from build123d import *
from OCP.BRepFilletAPI import BRepFilletAPI_MakeChamfer

# Parameters (mm, degrees)
SKETCH_1_R      = 1.55
EXTRUDE_1_DEPTH = 2.5
FILLET_1_R      = 10
CHAMFER_2_SIZE  = 0.615
CHAMFER_2_SIZE2 = 0.355070416


with BuildPart() as part:
    # 草图1 → 凸台-拉伸1 (new body)
    with BuildSketch(Plane(origin=(0, 0, 0), x_dir=(1, 0, 0), z_dir=(0, 1, 0))):
        with BuildLine():
            Line((47.899982554, 52.633397656), (59.52497064, 26.588251477))
            Line((59.52497064, 26.588251477), (85.869588061, 26.588251477))
            Line((85.869588061, 26.588251477), (94.505759306, 0))
            Line((94.505759306, 0), (85.869588061, -26.588251477))
            Line((85.869588061, -26.588251477), (59.52497064, -26.588251477))
            Line((59.52497064, -26.588251477), (47.899982554, -52.633397656))
            ThreePointArc((47.899982554, -52.633397656), (43.362068791, -56.315801292), (37.709796983, -54.831018053))
            ThreePointArc((37.709796983, -54.831018053), (34.400449937, -52.764318952), (30.978168019, -50.89055015))
            Line((30.978168019, -50.89055015), (-30.978168019, -50.89055015))
            ThreePointArc((-30.978168019, -50.89055015), (-34.400449937, -52.764318952), (-37.709796983, -54.831018053))
            ThreePointArc((-37.709796983, -54.831018053), (-43.362068791, -56.315801292), (-47.899982554, -52.633397656))
            Line((-47.899982554, -52.633397656), (-59.52497064, -26.588251477))
            Line((-59.52497064, -26.588251477), (-85.869588061, -26.588251477))
            Line((-85.869588061, -26.588251477), (-94.505759306, 0))
            Line((-94.505759306, 0), (-85.869588061, 26.588251477))
            Line((-85.869588061, 26.588251477), (-59.52497064, 26.588251477))
            Line((-59.52497064, 26.588251477), (-47.899982554, 52.633397656))
            ThreePointArc((-47.899982554, 52.633397656), (-43.362068791, 56.315801292), (-37.709796983, 54.831018053))
            ThreePointArc((-37.709796983, 54.831018053), (-34.400449937, 52.764318952), (-30.978168019, 50.89055015))
            Line((-30.978168019, 50.89055015), (30.978168019, 50.89055015))
            ThreePointArc((30.978168019, 50.89055015), (34.400449937, 52.764318952), (37.709796983, 54.831018053))
            ThreePointArc((37.709796983, 54.831018053), (43.362068791, 56.315801292), (47.899982554, 52.633397656))
        make_face()
        with Locations(Location((42, 50, 0), (0, 0, 270))):
            Circle(SKETCH_1_R, mode=Mode.SUBTRACT)
        with Locations(Location((42, -50, 0), (0, 0, 90))):
            Circle(SKETCH_1_R, mode=Mode.SUBTRACT)
        with Locations(Location((-42, -50, 0), (0, 0, 270))):
            Circle(SKETCH_1_R, mode=Mode.SUBTRACT)
        with Locations(Location((-42, 50, 0), (0, 0, 90))):
            Circle(SKETCH_1_R, mode=Mode.SUBTRACT)
        with Locations(Location((36, 43, 0), (0, 0, 270))):
            Circle(SKETCH_1_R, mode=Mode.SUBTRACT)
        with Locations(Location((32, -42, 0), (0, 0, 270))):
            Circle(SKETCH_1_R, mode=Mode.SUBTRACT)
        with Locations(Location((-32, -42, 0), (0, 0, 90))):
            Circle(SKETCH_1_R, mode=Mode.SUBTRACT)
        with Locations(Location((-36, 43, 0), (0, 0, 90))):
            Circle(SKETCH_1_R, mode=Mode.SUBTRACT)
        with Locations(Location((70.5, 9.435839055, 0), (0, 0, 270))):
            Circle(SKETCH_1_R, mode=Mode.SUBTRACT)
        with Locations(Location((70.5, -9.435839055, 0), (0, 0, 90))):
            Circle(SKETCH_1_R, mode=Mode.SUBTRACT)
        with Locations(Location((-70.5, -9.435839055, 0), (0, 0, 270))):
            Circle(SKETCH_1_R, mode=Mode.SUBTRACT)
        with Locations(Location((-70.5, 9.435839055, 0), (0, 0, 90))):
            Circle(SKETCH_1_R, mode=Mode.SUBTRACT)
        with Locations(Location((87.3, 0, 0), (0, 0, 270))):
            Circle(SKETCH_1_R, mode=Mode.SUBTRACT)
        with Locations(Location((-87.3, 0, 0), (0, 0, 90))):
            Circle(SKETCH_1_R, mode=Mode.SUBTRACT)
        with BuildLine():
            Line((77.169642998, -17.5), (77.169642998, 17.5))
            ThreePointArc((77.169642998, 17.5), (79.669642998, 20), (82.169642998, 17.5))
            Line((82.169642998, 17.5), (82.169642998, -17.5))
            ThreePointArc((82.169642998, -17.5), (79.669642998, -20), (77.169642998, -17.5))
        make_face(mode=Mode.SUBTRACT)
        with BuildLine():
            Line((-77.169642998, -17.5), (-77.169642998, 17.5))
            ThreePointArc((-77.169642998, 17.5), (-79.669642998, 20), (-82.169642998, 17.5))
            Line((-82.169642998, 17.5), (-82.169642998, -17.5))
            ThreePointArc((-82.169642998, -17.5), (-79.669642998, -20), (-77.169642998, -17.5))
        make_face(mode=Mode.SUBTRACT)
        with BuildLine():
            Line((-24.995975583, 14.429581723), (-10.56639386, 0))
            Line((-10.56639386, 0), (-24.995975583, -14.429581723))
            ThreePointArc((-24.995975583, -14.429581723), (-27.869597938, -17.042325553), (-30.978168019, -19.370614155))
            ThreePointArc((-30.978168019, -19.370614155), (-28.024295248, 0), (-30.978168019, 19.370614155))
            ThreePointArc((-30.978168019, 19.370614155), (-27.869597938, 17.042325553), (-24.995975583, 14.429581723))
        make_face(mode=Mode.SUBTRACT)
        with BuildLine():
            Line((14.429581723, 24.995975583), (0, 10.56639386))
            Line((0, 10.56639386), (-14.429581723, 24.995975583))
            ThreePointArc((-14.429581723, 24.995975583), (-17.042325553, 27.869597938), (-19.370614155, 30.978168019))
            ThreePointArc((-19.370614155, 30.978168019), (0, 28.024295248), (19.370614155, 30.978168019))
            ThreePointArc((19.370614155, 30.978168019), (17.042325553, 27.869597938), (14.429581723, 24.995975583))
        make_face(mode=Mode.SUBTRACT)
        with BuildLine():
            Line((24.995975583, -14.429581723), (10.56639386, 0))
            Line((10.56639386, 0), (24.995975583, 14.429581723))
            ThreePointArc((24.995975583, 14.429581723), (27.869597938, 17.042325553), (30.978168019, 19.370614155))
            ThreePointArc((30.978168019, 19.370614155), (28.024295248, 0), (30.978168019, -19.370614155))
            ThreePointArc((30.978168019, -19.370614155), (27.869597938, -17.042325553), (24.995975583, -14.429581723))
        make_face(mode=Mode.SUBTRACT)
        with BuildLine():
            Line((-14.429581723, -24.995975583), (0, -10.56639386))
            Line((0, -10.56639386), (14.429581723, -24.995975583))
            ThreePointArc((14.429581723, -24.995975583), (17.042325553, -27.869597938), (19.370614155, -30.978168019))
            ThreePointArc((19.370614155, -30.978168019), (0, -28.024295248), (-19.370614155, -30.978168019))
            ThreePointArc((-19.370614155, -30.978168019), (-17.042325553, -27.869597938), (-14.429581723, -24.995975583))
        make_face(mode=Mode.SUBTRACT)
        with BuildLine():
            Line((41.468701347, -26.829343455), (41.468701347, 26.829343455))
            ThreePointArc((41.468701347, 26.829343455), (44.919200659, 30.279842767), (48.36969997, 26.829343455))
            Line((48.36969997, 26.829343455), (48.36969997, -26.829343455))
            ThreePointArc((48.36969997, -26.829343455), (44.919200659, -30.279842767), (41.468701347, -26.829343455))
        make_face(mode=Mode.SUBTRACT)
        with BuildLine():
            Line((-26.453510137, -34.636976429), (26.453510137, -34.636976429))
            ThreePointArc((26.453510137, -34.636976429), (29.060662927, -37.244129219), (26.453510137, -39.851282009))
            Line((26.453510137, -39.851282009), (-26.453510137, -39.851282009))
            ThreePointArc((-26.453510137, -39.851282009), (-29.060662927, -37.244129219), (-26.453510137, -34.636976429))
        make_face(mode=Mode.SUBTRACT)
        with BuildLine():
            Line((-26.453510137, 34.636976429), (26.453510137, 34.636976429))
            ThreePointArc((26.453510137, 34.636976429), (29.060662927, 37.244129219), (26.453510137, 39.851282009))
            Line((26.453510137, 39.851282009), (-26.453510137, 39.851282009))
            ThreePointArc((-26.453510137, 39.851282009), (-29.060662927, 37.244129219), (-26.453510137, 34.636976429))
        make_face(mode=Mode.SUBTRACT)
        with BuildLine():
            Line((-41.468701347, -26.829343455), (-41.468701347, 26.829343455))
            ThreePointArc((-41.468701347, 26.829343455), (-44.919200659, 30.279842767), (-48.36969997, 26.829343455))
            Line((-48.36969997, 26.829343455), (-48.36969997, -26.829343455))
            ThreePointArc((-48.36969997, -26.829343455), (-44.919200659, -30.279842767), (-41.468701347, -26.829343455))
        make_face(mode=Mode.SUBTRACT)
    extrude(amount=EXTRUDE_1_DEPTH)

    # 圆角1
    fillet_1_edges = [part.edges().sort_by_distance(p)[0] for p in [
        (59.52497064, 1.25, -26.588251477),
        (85.869588061, 1.25, -26.588251477),
        (94.505759306, 1.25, 0),
        (85.869588061, 1.25, 26.588251477),
        (59.52497064, 1.25, 26.588251477),
        (30.978168019, 1.25, 50.89055015),
        (-30.978168019, 1.25, 50.89055015),
        (-59.52497064, 1.25, 26.588251477),
        (-85.869588061, 1.25, 26.588251477),
        (-94.505759306, 1.25, 0),
        (-85.869588061, 1.25, -26.588251477),
        (-59.52497064, 1.25, -26.588251477),
        (-30.978168019, 1.25, -50.89055015),
        (30.978168019, 1.25, -50.89055015),
    ]]
    fillet(fillet_1_edges, radius=FILLET_1_R)

    # 倒角2: one chamfer whose edges measure the first distance from different faces: ONE call of the kernel's chamfer builder (chamfer() names one face for all edges)
    chamfer_2_edges_1 = [part.edges().sort_by_distance(p)[0] for p in [
        (70.5, 0, 10.985839055),
    ]]
    chamfer_2_side_1 = [part.faces().sort_by_distance(p)[0] for p in [
        (70.5, 1.25, 10.985839055),
    ]]
    chamfer_2_edges_2 = [part.edges().sort_by_distance(p)[0] for p in [
        (-70.5, 0, 7.885839055),
    ]]
    chamfer_2_side_2 = [part.faces().sort_by_distance(p)[0] for p in [
        (-70.5, 1.25, 7.885839055),
    ]]
    chamfer_2_edges_3 = [part.edges().sort_by_distance(p)[0] for p in [
        (70.5, 0, -10.985839055),
    ]]
    chamfer_2_side_3 = [part.faces().sort_by_distance(p)[0] for p in [
        (70.5, 1.25, -10.985839055),
    ]]
    chamfer_2_edges_4 = [part.edges().sort_by_distance(p)[0] for p in [
        (-70.5, 0, -7.885839055),
    ]]
    chamfer_2_side_4 = [part.faces().sort_by_distance(p)[0] for p in [
        (-70.5, 1.25, -7.885839055),
    ]]
    chamfer_2_edges_5 = [part.edges().sort_by_distance(p)[0] for p in [
        (87.3, 0, -1.55),
    ]]
    chamfer_2_side_5 = [part.faces().sort_by_distance(p)[0] for p in [
        (87.3, 1.25, -1.55),
    ]]
    chamfer_2_edges_6 = [part.edges().sort_by_distance(p)[0] for p in [
        (-87.3, 0, 1.55),
    ]]
    chamfer_2_side_6 = [part.faces().sort_by_distance(p)[0] for p in [
        (-87.3, 1.25, 1.55),
    ]]
    chamfer_2_edges_7 = [part.edges().sort_by_distance(p)[0] for p in [
        (-42, 0, 48.45),
    ]]
    chamfer_2_side_7 = [part.faces().sort_by_distance(p)[0] for p in [
        (-42, 1.25, 48.45),
    ]]
    chamfer_2_edges_8 = [part.edges().sort_by_distance(p)[0] for p in [
        (-42, 0, -48.45),
    ]]
    chamfer_2_side_8 = [part.faces().sort_by_distance(p)[0] for p in [
        (-42, 1.25, -48.45),
    ]]
    chamfer_2_edges_9 = [part.edges().sort_by_distance(p)[0] for p in [
        (42, 0, -51.55),
    ]]
    chamfer_2_side_9 = [part.faces().sort_by_distance(p)[0] for p in [
        (42, 1.25, -51.55),
    ]]
    chamfer_2_edges_10 = [part.edges().sort_by_distance(p)[0] for p in [
        (42, 0, 51.55),
    ]]
    chamfer_2_side_10 = [part.faces().sort_by_distance(p)[0] for p in [
        (42, 1.25, 51.55),
    ]]
    chamfer_2 = BRepFilletAPI_MakeChamfer(part.part.solid().wrapped)
    for e in chamfer_2_edges_1:
        chamfer_2.Add(CHAMFER_2_SIZE, CHAMFER_2_SIZE2, e.wrapped, chamfer_2_side_1[0].wrapped)  # the first distance lies on this face
    for e in chamfer_2_edges_2:
        chamfer_2.Add(CHAMFER_2_SIZE, CHAMFER_2_SIZE2, e.wrapped, chamfer_2_side_2[0].wrapped)  # the first distance lies on this face
    for e in chamfer_2_edges_3:
        chamfer_2.Add(CHAMFER_2_SIZE, CHAMFER_2_SIZE2, e.wrapped, chamfer_2_side_3[0].wrapped)  # the first distance lies on this face
    for e in chamfer_2_edges_4:
        chamfer_2.Add(CHAMFER_2_SIZE, CHAMFER_2_SIZE2, e.wrapped, chamfer_2_side_4[0].wrapped)  # the first distance lies on this face
    for e in chamfer_2_edges_5:
        chamfer_2.Add(CHAMFER_2_SIZE, CHAMFER_2_SIZE2, e.wrapped, chamfer_2_side_5[0].wrapped)  # the first distance lies on this face
    for e in chamfer_2_edges_6:
        chamfer_2.Add(CHAMFER_2_SIZE, CHAMFER_2_SIZE2, e.wrapped, chamfer_2_side_6[0].wrapped)  # the first distance lies on this face
    for e in chamfer_2_edges_7:
        chamfer_2.Add(CHAMFER_2_SIZE, CHAMFER_2_SIZE2, e.wrapped, chamfer_2_side_7[0].wrapped)  # the first distance lies on this face
    for e in chamfer_2_edges_8:
        chamfer_2.Add(CHAMFER_2_SIZE, CHAMFER_2_SIZE2, e.wrapped, chamfer_2_side_8[0].wrapped)  # the first distance lies on this face
    for e in chamfer_2_edges_9:
        chamfer_2.Add(CHAMFER_2_SIZE, CHAMFER_2_SIZE2, e.wrapped, chamfer_2_side_9[0].wrapped)  # the first distance lies on this face
    for e in chamfer_2_edges_10:
        chamfer_2.Add(CHAMFER_2_SIZE, CHAMFER_2_SIZE2, e.wrapped, chamfer_2_side_10[0].wrapped)  # the first distance lies on this face
    add(Compound.cast(chamfer_2.Shape()), mode=Mode.REPLACE)


solid = part.part
Design review of the part built by this model. Coordinates are the model's own, in mm. A direction names the side the tool comes from. Give positions to 0.01 mm unless a question says otherwise; leave off trailing zeros. Return JSON: item names as keys, results as strings. Group by question number.
Item 1: Clearance check with flat-ended pins moving along their axes: pin 1 Ø0.8 at (y, z) = (2, 6) entering from -X; pin 2 Ø1.9 at (x, z) = (42, 50) entering from -Y; pin 3 Ø3.5 at (x, z) = (70.5, -9.44) entering from -Y; pin 4 Ø1 at (y, z) = (1, -1) entering from -X. State where each tip first meets the part, or that it passes through.
Item 2: Take a section at A-A (y = 1.7). Count the separate pieces of the cut face and the enclosed holes in it, plus the area to 3 significant figures.
Item 3: The part is to be moulded in two halves that separate along X. For faces 1 (the flat face through (1, 0, -1)), 2 (the cylindrical face through (-60.638, 1.268, 28.155)), 3 (the cylindrical face through (-45, 1.23, 30.28)), 4 (the flat face through (90.77, 1.23, -11.5)), say which applies: pulls with the +X half, pulls with the -X half, needs draft (parallel to the pull), parting line crosses it, or undercut.
Item 4: Wall thickness on line 1 along X through (y, z) = (2, -43); line 2 along X through (y, z) = (2, 50); line 3 along Z through (x, y) = (4, 0.1): over which ranges is each line inside the solid? List them lowest first.
Item 5: Tool access review of faces 5 (the cylindrical face through (-84.55, 1.27, 24.63)), 6 (the cylindrical face through (44.84, 1.23, -30.28)): name each direction out of +Z, -Z, +X, -X, +Y, -Y from which nothing blocks a thin tool from reaching the whole face with its end or side.
Return value:
{
 "1": {"pin 1": "stops at x = -92.69", "pin 2": "passes through", "pin 3": "stops at y = 0.26", "pin 4": "stops at x = -93.98"},
 "2": {"separate pieces": "1", "enclosed holes": "24", "area": "11,800 mm2"},
 "3": {"face 1": "needs draft", "face 2": "pulls with the -X half", "face 3": "undercut", "face 4": "pulls with the +X half"},
 "4": {"line 1": "x = -52.2 to -37.55, -34.45 to 34.45, 37.55 to 52.2", "line 2": "x = -49.08 to -43.55, -40.45 to 40.45, 43.55 to 49.08", "line 3": "z = -50.89 to -39.85, -34.64 to -28.15, -14.57 to 14.57, 28.15 to 34.64, 39.85 to 50.89"},
 "5": {"face 5": "+Z, -X, +Y, -Y", "face 6": "+Y, -Y"}
}
